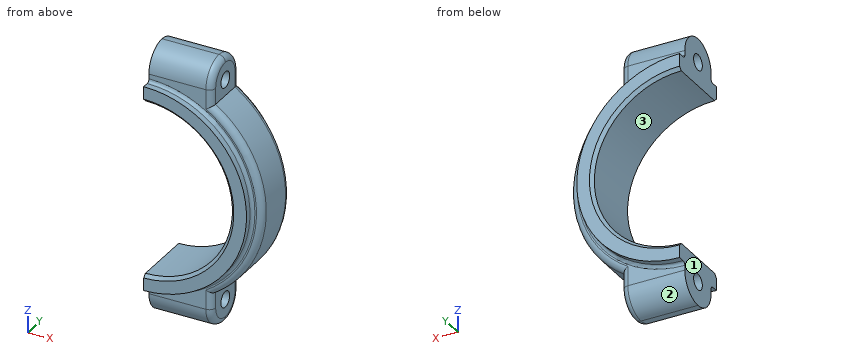
Autodesk Inventor part; units mm, degrees
ref_plane "YZ Plane" through (0, 0, 0) normal (1, 0, 0) x (0, 1, 0)
ref_plane "XZ Plane" through (0, 0, 0) normal (0, 1, 0) x (-1, 0, 0)
ref_plane "XY Plane" through (0, 0, 0) normal (0, 0, 1) x (1, 0, 0)
sketch "Sketch1" plane through (0, 0, 0) normal (0, 1, 0) x (-1, 0, 0)
  arc A0 (0, 27.5) -> (0, -27.5) centre (0, 0) ccw
  arc A1 (0, 32.5) -> (0, -32.5) centre (0, 0) ccw
  line L0 (0, -32.5) -> (0, -42.5)
  line L1 (0, -42.5) -> (-20, -42.5)
  line L2 (-20, -42.5) -> (-20, -25.6174)
  line L3 (-20, 25.6174) -> (-20, 42.5)
  line L4 (-20, 42.5) -> (0, 42.5)
  line L5 (0, 42.5) -> (0, 32.5)
  line L6 (0, -32.5) -> (0, -27.5)
  line L7 (0, 27.5) -> (0, 32.5)
  arc A2 (-20, 29.9333) -> (-20, -29.9333) centre (0, 0) ccw
  dimension "d0" = 27.5
  dimension "d1" = 32.5
  dimension "d2" = 10
  dimension "d3" = 20
  dimension "d4" = 36
extrude "Extrusion1" add sketch "Sketch1" along normal mid plane 21 contours A0 L6 A1 L7
extrude "Extrusion2" add sketch "Sketch1" along normal mid plane 15 contours A1 L3 L4 L5 | L0 L1 L2 A1 | A1 L2 A2 L3
sketch "Sketch2" plane through (0, -10.5, -27.5) normal (-1, 0, 0) x (0, 0, 1)
  line L0 (0, 21) -> (0, 0)
  line L1 (55, 0) -> (55, 21)
  point P0 (27.5, 10.5)
  point P1 (-7.5, 10.5)
  point P2 (62.5, 10.5)
  dimension "d9" = 7.5
  dimension "d10" = 7.5
hole "Hole1" at (0, 0, -35) at (0, 0, 35) direction (1, 0, 0) diameter 5 end through all
full round fillet "Full Round Fillet1" first side at (9.2593, 7.5, 38.8519) centre faces at (13.3333, -2.5, -42.5) second side at (9.2593, -7.5, 38.8519)
full round fillet "Full Round Fillet2" first side at (9.2593, -7.5, 38.8519) centre faces at (6.6667, -2.5, 42.5) second side at (9.2593, 7.5, 38.8519)
fillet "Fillet1" radius 2 10 edges at (36, -7.5, 0) (20, 5.3033, 40.3033) (20, -5.3033, 40.3033) (20, 7.5, 32.4667) (20, -7.5, 32.4667) (36, 7.5, 0) (20, -7.5, -32.4667) (20, 7.5, -32.4667) (20, 5.3033, -40.3033) (20, -5.3033, -40.3033)
chamfer "Chamfer1" distance 1 angle 45 2 edges at (27.5, -10.5, 0) (27.5, 10.5, 0)
fillet "Fillet2" radius 1 2 edges at (32.5, 7.5, 0) (32.5, -7.5, 0)
properties part number "Pokrywa stopy korbowodu"
Source: CAD feature listing. Evaluate the final solid. Frame: model axes, mm. Face numbers are marked on the shaded views. Coordinates: 2 decimals unless noted, no trailing zeros. Loops run counter-clockwise (first coordinate to the right, second up) from the corner with the lowest first, then second, coordinate; pieces in that order, holes last. Notation, with made-up numbers: (32, 16.5) -> (48, 16.5) arc R15 ccw to (48, 32.5) -> close; hole circle Ø6 at (72, -15.75). An arc over 180 degrees is marked (long way). Answer in a Markdown table with one row per item. Add a question column.
Q1. Ray query, line 1 along Y through (x, z) = (10, 35); line 2 along Z through (x, y) = (12.75, 0); line 3 along Z through (x, y) = (13.75, 0). Return the intervals inside material, ascending.
Q2. Section A-A on z = 0. Return the cut outline in (x, y).
Q3. Pull-direction query (Z, two-part tool) for the marked faces 1, 2 and 3; classes: pulls with the +Z half, pulls with the -Z half, needs draft (parallel to the pull), parting line crosses it, or undercut.
Q4. Contact query for flat-ended pins moving along their axis: pin 1 Ø6 at (x, y) = (5, -5) entering from -Z; pin 2 Ø1.5 at (y, z) = (5, 18) entering from -X; pin 3 Ø3 at (x, z) = (21.5, -28.5) entering from -Y. Output: stop coordinate, or through.
Q5. Section B-B on x = 9. Give the number of separate pieces and of enclosed holes in the cut face, and give its area (3 significant figures).
Computed values:
| question | item | result |
|---|---|---|
| 1 | line 1 | y = -7.5 to -2.5, 2.5 to 7.5 |
| 1 | line 2 | z = -42.5 to -37.5, -32.5 to -24.37, 24.37 to 32.5, 37.5 to 42.5 |
| 1 | line 3 | z = -42.5 to -37.5, -32.5 to -23.82, 23.82 to 32.5, 37.5 to 42.5 |
| 2 | outline | (27.5, -9.5) -> (28.5, -10.5) -> (32.5, -10.5) -> (32.5, -8.5) arc R1 cw to (33.5, -7.5) -> (34, -7.5) arc R2 ccw to (36, -5.5) -> (36, 5.5) arc R2 ccw to (34, 7.5) -> (33.5, 7.5) arc R1 cw to (32.5, 8.5) -> (32.5, 10.5) -> (28.5, 10.5) -> (27.5, 9.5) -> close |
| 3 | face 1 | needs draft |
| 3 | face 2 | pulls with the -Z half |
| 3 | face 3 | undercut |
| 4 | pin 1 | stops at z = -42.23 |
| 4 | pin 2 | stops at x = 20.12 |
| 4 | pin 3 | stops at y = -7.49 |
| 5 | separate pieces | 2 |
| 5 | enclosed holes | 2 |
| 5 | area | 470 mm^2 |
